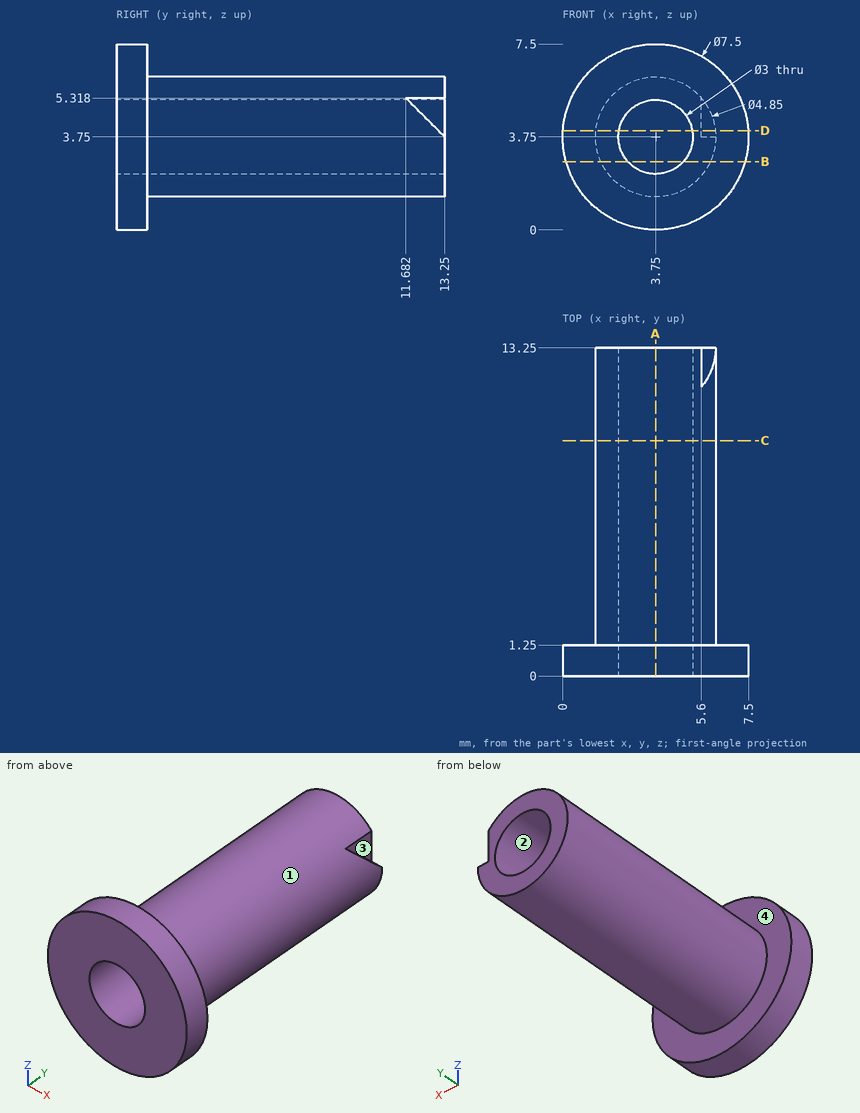
The drawing under review shows one solid part. Ordinate dimensions are in mm from its lowest x, y, z. Round coordinates to 2 decimals unless told otherwise and drop trailing zeros. Loops run counter-clockwise (first coordinate to the right, second up) from the corner with the lowest first, then second, coordinate; pieces in that order, holes last. Notation, with made-up numbers: (7.5, 60.5) -> (52.5, 60.5) arc R18 ccw to (52.5, 95.5) -> close; hole circle Ø3 at (27, 14.5). An arc over 180 degrees is marked (long way). Answer in a Markdown table with one row per item.
1) Consider section A-A, the plane x = 3.75. Write out the cut boundary in (y, z) (3 decimals), plus the area to 3 significant figures.
Taken from the geometry:
| item | result |
|---|---|
| outline | (0, 0) -> (1.25, 0) -> (1.25, 1.325) -> (13.25, 1.325) -> (13.25, 2.25) -> (0, 2.25) -> close; (0, 5.25) -> (13.25, 5.25) -> (13.25, 6.175) -> (1.25, 6.175) -> (1.25, 7.5) -> (0, 7.5) -> close |
| area | 27.8 mm² |
2) Draft analysis for pull direction X (two halves, no side actions). For the marked faces 1, 2, 3 and 4, state which applies: pulls with the +X half, pulls with the -X half, needs draft (parallel to the pull), parting line crosses it, or undercut.
Taken from the geometry:
| item | result |
|---|---|
| face 1 | parting line crosses it |
| face 2 | undercut |
| face 3 | pulls with the +X half |
| face 4 | needs draft |
3) Consider section C-C, the plane y = 9.5. Write out the cut boundary in (x, z) (3 decimals).
Taken from the geometry:
| item | result |
|---|---|
| outline | circle Ø4.85 at (3.75, 3.75); hole circle Ø3 at (3.75, 3.75) |
4) Consider section D-D, the plane z = 4. Write out the cut boundary in (x, y), plus the area to 3 significant figures.
Taken from the geometry:
| item | result |
|---|---|
| outline | (0.01, 0) -> (2.27, 0) -> (2.27, 13.25) -> (1.34, 13.25) -> (1.34, 1.25) -> (0.01, 1.25) -> close; (5.23, 0) -> (7.49, 0) -> (7.49, 1.25) -> (6.16, 1.25) -> (6.16, 13) -> (5.6, 13) -> (5.6, 13.25) -> (5.23, 13.25) -> close |
| area | 27.9 mm² |
5) Wall thickness on line 1 along Z through (x, y) = (3.75, 10) (3 decimals); line 2 along Y through (x, z) = (4.25, 7); line 3 along X through (y, z) = (4.5, 4.25): over which ranges is each line inside the solid? List them lowest first.
Taken from the geometry:
| item | result |
|---|---|
| line 1 | z = 1.325 to 2.25, 5.25 to 6.175 |
| line 2 | y = 0 to 1.25 |
| line 3 | x = 1.38 to 2.34, 5.16 to 6.12 |
6) Consider section B-B, the plane z = 2.75. Write out the cut boundary in (x, y), plus the area to 3 significant figures.
Taken from the geometry:
| item | result |
|---|---|
| outline | (0.14, 0) -> (2.63, 0) -> (2.63, 13.25) -> (1.54, 13.25) -> (1.54, 1.25) -> (0.14, 1.25) -> close; (4.87, 0) -> (7.36, 0) -> (7.36, 1.25) -> (5.96, 1.25) -> (5.96, 13.25) -> (4.87, 13.25) -> close |
| area | 32.4 mm² |
7) For pin 1 Ø1.3 at (y, z) = (12.5, 4.5) entering from +X; pin 2 Ø1.5 at (y, z) = (5.5, 6) entering from -X (1 decimal); pin 3 Ø2 at (x, y) = (4, 3.5) entering from -Z (3 decimals), all flat-tipped, find the tip position at first contact; note any pin that passes through.
Taken from the geometry:
| item | result |
|---|---|
| pin 1 | stops at x = 6.17 |
| pin 2 | stops at x = 1.8 |
| pin 3 | stops at z = 1.325 |
